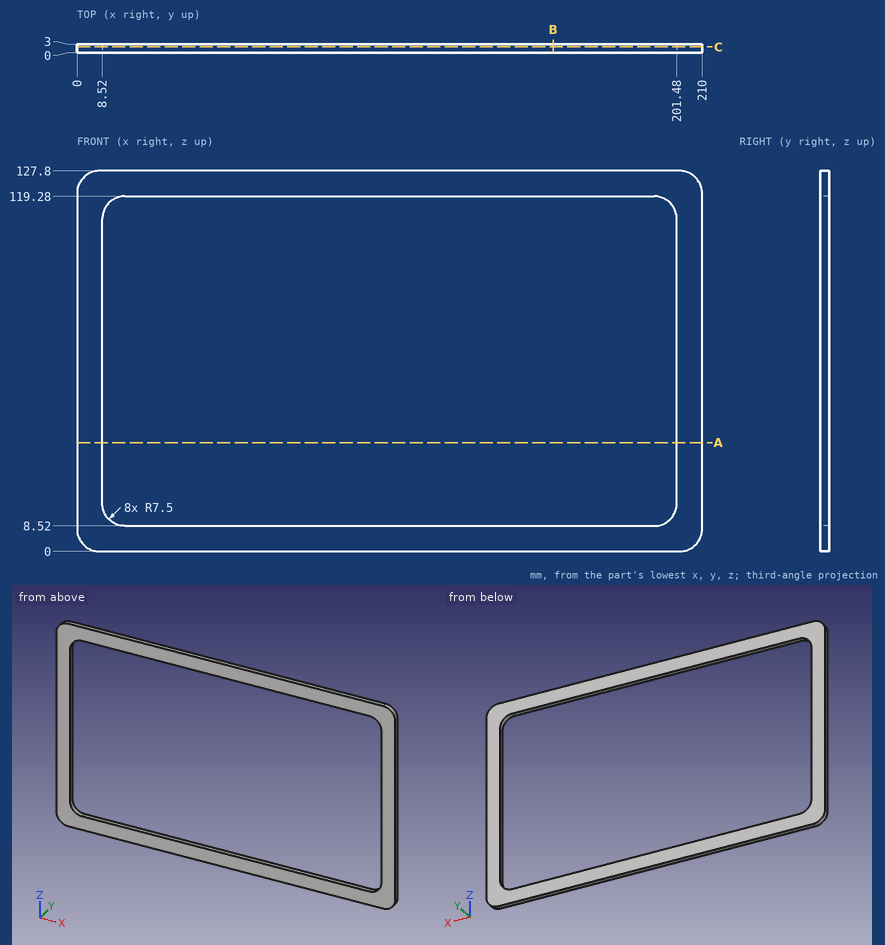
Here's the drawing with two shaded views (mm, measured from the low corner). I have some questions. Give positions to 0.01 mm unless a question says otherwise; leave off trailing zeros. Write each loop counter-clockwise with the first axis right and the second up, starting at its lowest first coordinate (ties: lowest second). Pieces come first, ordered by that corner, then holes. Notation, with made-up numbers: (47.25, 4) -> (58.25, 4) arc R5 cw to (58.25, 8) -> close; hole circle Ø2 at (6.25, 39). An arc over 180 degrees is marked (long way). One line per item, written item: value.
Q1. Imagine slicing it at B-B on x = 160. Please give me the cut outline in (y, z).
Results found:
outline: (0, 0) -> (3, 0) -> (3, 8.52) -> (0, 8.52) -> close; (0, 119.28) -> (3, 119.28) -> (3, 127.8) -> (0, 127.8) -> close
Q2. Imagine slicing it at A-A on z = 36.5. Please give me the cut outline in (x, y), and give its area (3 significant figures).
Results found:
outline: (0, 0) -> (8.52, 0) -> (8.52, 3) -> (0, 3) -> close; (201.48, 0) -> (210, 0) -> (210, 3) -> (201.48, 3) -> close
area: 51.1 mm^2
Q3. Imagine slicing it at C-C on y = 2. Please give me the cut outline in (x, z), and give its area (3 significant figures).
Results found:
outline: (0, 7.5) arc R7.5 ccw to (7.5, 0) -> (202.5, 0) arc R7.5 ccw to (210, 7.5) -> (210, 120.3) arc R7.5 ccw to (202.5, 127.8) -> (7.5, 127.8) arc R7.5 ccw to (0, 120.3) -> close; hole (8.52, 16.02) arc R7.5 ccw to (16.02, 8.52) -> (193.98, 8.52) arc R7.5 ccw to (201.48, 16.02) -> (201.48, 111.78) arc R7.5 ccw to (193.98, 119.28) -> (16.02, 119.28) arc R7.5 ccw to (8.52, 111.78) -> close
area: 5,470 mm^2
Q4. Please list where these lines run through material, in increasing order: line 1 (X direction, y = 1.2, z = 98.5); line 2 (Z direction, x = 64, y = 1.55); line 3 (X direction, y = 1.4, z = 121). Write a range as [from, to].
Results found:
line 1: x = [0, 8.52], [201.48, 210]
line 2: z = [0, 8.52], [119.28, 127.8]
line 3: x = [0.03, 209.97]
